```python
from build123d import *

# Parameters (mm, degrees)
SKETCH26_R          = 2.05
SKETCH26_R_2        = 2.15
SKETCH26_R_3        = 4
SKETCH26_R_4        = 1.27
SKETCH26_R_5        = 2.141312715
BOSS_EXTRUDE4_DEPTH = 2


with BuildPart() as part:
    # Sketch26 → Boss-Extrude4 (new body)
    with BuildSketch(Plane(origin=(0, 0, 0), x_dir=(1, 0, 0), z_dir=(0, 1, 0))):
        with BuildLine():
            Line((75.767236042, 90.766820858), (50.767236042, 90.766820858))
            Line((50.767236042, 90.766820858), (-51.032763958, 90.766820858))
            Line((-51.032763958, 90.766820858), (-76.278800323, 90.766820858))
            Line((-76.278800323, 90.766820858), (-115.954777141, 90.766820858))
            ThreePointArc((-115.954777141, 90.766820858), (-117.722544094, 90.034587811), (-118.454777141, 88.266820858))
            Line((-118.454777141, 88.266820858), (-118.454777141, 33.266820858))
            ThreePointArc((-118.454777141, 33.266820858), (-117.722544094, 31.499053905), (-115.954777141, 30.766820858))
            Line((-115.954777141, 30.766820858), (-76.278800323, 30.766820858))
            Line((-76.278800323, 30.766820858), (-51.571443107, -49.270587217))
            ThreePointArc((-51.571443107, -49.270587217), (-50.667003064, -50.544835199), (-49.182671596, -51.033179142))
            Line((-49.182671596, -51.033179142), (48.917143681, -51.033179142))
            ThreePointArc((48.917143681, -51.033179142), (50.404299167, -50.542748389), (51.307977226, -49.26387399))
            Line((51.307977226, -49.26387399), (75.767236042, 30.766820858))
            Line((75.767236042, 30.766820858), (115.443212861, 30.766820858))
            ThreePointArc((115.443212861, 30.766820858), (117.210979814, 31.499053905), (117.943212861, 33.266820858))
            Line((117.943212861, 33.266820858), (117.943212861, 88.266820858))
            ThreePointArc((117.943212861, 88.266820858), (117.210979814, 90.034587811), (115.443212861, 90.766820858))
            Line((115.443212861, 90.766820858), (75.767236042, 90.766820858))
        make_face()
        with Locations((-45.02, -45.02)):
            Circle(SKETCH26_R, mode=Mode.SUBTRACT)
        with Locations((-4.845188419, -22.879546923)):
            Circle(SKETCH26_R_2, mode=Mode.SUBTRACT)
        with Locations((45.02, -45.02)):
            Circle(SKETCH26_R, mode=Mode.SUBTRACT)
        with Locations((4.954811581, -22.879546923)):
            Circle(SKETCH26_R_2, mode=Mode.SUBTRACT)
        with BuildLine():
            Line((-13.610657589, 22.45), (-0.75, 22.45))
            Line((-0.75, 22.45), (-0.75, 26.95))
            Line((-0.75, 26.95), (0.75, 26.95))
            Line((0.75, 26.95), (0.75, 22.45))
            Line((0.75, 22.45), (10, 22.45))
            Line((10, 22.45), (13.610657589, 22.45))
            ThreePointArc((13.610657589, 22.45), (17.325300122, 8.983428358), (10, -2.911406616))
            Line((10, -2.911406616), (10, -18.55))
            Line((10, -18.55), (0.75, -18.55))
            Line((0.75, -18.55), (0.75, -23.05))
            Line((0.75, -23.05), (-0.75, -23.05))
            Line((-0.75, -23.05), (-0.75, -18.55))
            Line((-0.75, -18.55), (-10, -18.55))
            Line((-10, -18.55), (-10, -2.911406616))
            ThreePointArc((-10, -2.911406616), (-17.325300122, 8.983428358), (-13.610657589, 22.45))
        make_face(mode=Mode.SUBTRACT)
        with Locations((-103.332763958, 45.766820858)):
            Circle(SKETCH26_R_3, mode=Mode.SUBTRACT)
        with BuildLine():
            ThreePointArc((-75.528800323, 39.191107079), (-76.278800323, 38.441107079), (-77.028800323, 39.191107079))
            Line((-77.028800323, 39.191107079), (-77.028800323, 51.691107079))
            ThreePointArc((-77.028800323, 51.691107079), (-76.278800323, 52.441107079), (-75.528800323, 51.691107079))
            Line((-75.528800323, 51.691107079), (-75.528800323, 39.191107079))
        make_face(mode=Mode.SUBTRACT)
        with Locations((-4.845188419, 26.779546923)):
            Circle(SKETCH26_R_2, mode=Mode.SUBTRACT)
        with Locations((-45.02, 45.02)):
            Circle(SKETCH26_R, mode=Mode.SUBTRACT)
        with Locations((-103.332763958, 65.066820858)):
            Circle(SKETCH26_R_4, mode=Mode.SUBTRACT)
        with Locations((-103.332763958, 75.266820858)):
            Circle(SKETCH26_R_5, mode=Mode.SUBTRACT)
        with Locations((-103.332763958, 85.466820858)):
            Circle(SKETCH26_R_4, mode=Mode.SUBTRACT)
        with BuildLine():
            ThreePointArc((-77.028800323, 81.095149015), (-76.278800323, 81.845149015), (-75.528800323, 81.095149015))
            Line((-75.528800323, 81.095149015), (-75.528800323, 68.595149015))
            ThreePointArc((-75.528800323, 68.595149015), (-76.278800323, 67.845149015), (-77.028800323, 68.595149015))
            Line((-77.028800323, 68.595149015), (-77.028800323, 81.095149015))
        make_face(mode=Mode.SUBTRACT)
        with Locations((-81.132763958, 75.266820858)):
            Circle(SKETCH26_R_4, mode=Mode.SUBTRACT)
        with Locations((4.954811581, 26.779546923)):
            Circle(SKETCH26_R_2, mode=Mode.SUBTRACT)
        with Locations((45.02, 45.02)):
            Circle(SKETCH26_R, mode=Mode.SUBTRACT)
        with BuildLine():
            Line((76.763272408, 51.691107079), (76.763272408, 39.191107079))
            ThreePointArc((76.763272408, 39.191107079), (76.013272408, 38.441107079), (75.263272408, 39.191107079))
            Line((75.263272408, 39.191107079), (75.263272408, 51.691107079))
            ThreePointArc((75.263272408, 51.691107079), (76.013272408, 52.441107079), (76.763272408, 51.691107079))
        make_face(mode=Mode.SUBTRACT)
        with Locations((103.067236042, 45.766820858)):
            Circle(SKETCH26_R_3, mode=Mode.SUBTRACT)
        with Locations((103.067236042, 65.066820858)):
            Circle(SKETCH26_R_4, mode=Mode.SUBTRACT)
        with BuildLine():
            Line((75.263272408, 68.595149015), (75.263272408, 81.095149015))
            ThreePointArc((75.263272408, 81.095149015), (76.013272408, 81.845149015), (76.763272408, 81.095149015))
            Line((76.763272408, 81.095149015), (76.763272408, 68.595149015))
            ThreePointArc((76.763272408, 68.595149015), (76.013272408, 67.845149015), (75.263272408, 68.595149015))
        make_face(mode=Mode.SUBTRACT)
        with Locations((80.867236042, 75.266820858)):
            Circle(SKETCH26_R_4, mode=Mode.SUBTRACT)
        with Locations((103.067236042, 75.266820858)):
            Circle(SKETCH26_R_5, mode=Mode.SUBTRACT)
        with Locations((103.067236042, 85.466820858)):
            Circle(SKETCH26_R_4, mode=Mode.SUBTRACT)
    extrude(amount=BOSS_EXTRUDE4_DEPTH)


solid = part.part
```
Here's how the part is built. I have some questions about the finished solid (model axes, mm). A direction names the side the tool comes from. Coordinates: 2 decimals unless noted, no trailing zeros. Order: outer loops, then holes, each group sorted by start corner. A loop starts at its lowest first (then second) coordinate and runs counter-clockwise, first axis right, second up. Notation, with made-up numbers: (51.25, -32.5) -> (70.25, -32.5) arc R16 ccw to (70.25, -23.5) -> close; hole circle Ø4 at (5.5, -32.75). An arc over 180 degrees is marked (long way). Return JSON: item names as keys, results as strings.
1) If we section it at D-D on y = 1.15: State how many separate pieces and enclosed holes the cut face has, plus the area to 3 significant figures.
Conclusion:
{"separate pieces": "1", "enclosed holes": "23", "area": "23,100 mm²"}
2) If we section it at B-B on x = 56: List the corners of the cut face in (y, z) for me, plus the area to 3 significant figures.
Conclusion:
{"outline": "(0, -90.77) -> (2, -90.77) -> (2, 33.91) -> (0, 33.91) -> close", "area": "249 mm²"}
3) If we section it at C-C on z = 29.5: List the corners of the cut face in (x, y) for me.
Conclusion:
{"outline": "(-57.67, 0) -> (57.35, 0) -> (57.35, 2) -> (-57.67, 2) -> close"}
4) If I drill on probe 1 along X at (y, z) = (1.5, -78); probe 2 along Z at (x, y) = (76, 1.7); probe 3 along Z at (x, y) = (45.02, 0.6), over which ranges is the centre line in solid material (lowest first)?
Conclusion:
{"probe 1": "x = -118.45 to -77.03, -75.53 to 75.26, 76.76 to 117.94", "probe 2": "z = -90.77 to -81.85, -67.85 to -52.44, -38.44 to -30.77", "probe 3": "z = -90.77 to -47.07, -42.97 to 42.97, 47.07 to 51.03"}
5) On a 3-axis mill with a long thin cutter (end or side, diameter ignored), from which of +Z, -Z, +X, -X, +Y, -Y can I reach the whole of each face in a straight line? I mean faces 5 (the cylindrical face through (-17.3, 1, -8.8)), 6 (the flat face through (-2, 2, -37)). Say none if no direction works.
Conclusion:
{"face 5": "+Y, -Y", "face 6": "+Z, -Z, +X, -X, +Y"}
6) If we section it at A-A on z = -20: List the corners of the cut face in (x, y) for me.
Conclusion:
{"outline": "(-72.96, 0) -> (-15.27, 0) -> (-15.27, 2) -> (-72.96, 2) -> close; (15.27, 0) -> (72.48, 0) -> (72.48, 2) -> (15.27, 2) -> close"}
7) Thinking about a two-plate mould opening in Z: for faces 1 (the cylindrical face through (-2.86, 0.99, 23.7)), 2 (the flat face through (-2, 0, -37)), 3 (the flat face through (63.366, 0.986, 9.809)), 4 (the cylindrical face through (101.489, 0.986, -76.714)), which applies, +Z half, -Z half, draft (parallel to the pull), parting line (faces both ways), or undercut?
Conclusion:
{"face 1": "undercut", "face 2": "draft", "face 3": "+Z half", "face 4": "undercut"}
8) I'm going to push flat-ended pins straight in: P1, Ø1, axis at y = 1.5, z = 20.5, coming from the +X side; P2, Ø5, axis at x = -16, z = 4, coming from the -Y side; P3, Ø5, axis at x = -103.33, z = -45.77, coming from the +Y side. Where does each tip first touch, or does it pass through?
Conclusion:
{"P1": "stops at x = 60.25", "P2": "stops at y = 0", "P3": "passes through"}
